For this review, take the finished solid that the model builds, in its own axes (mm). Face numbers are marked on the shaded views. A direction names the side the tool comes from. Give positions to 0.01 mm unless a question says otherwise; leave off trailing zeros. Loops run counter-clockwise (first coordinate to the right, second up) from the corner with the lowest first, then second, coordinate; pieces in that order, holes last. Notation, with made-up numbers: (66, 54.5) -> (113, 54.5) arc R12 cw to (113, 63.5) -> close; hole circle Ø2 at (66, -39). An arc over 180 degrees is marked (long way). Answer as CSV lines item,"result". Start each with the question number.
Item 1: Clearance check with a flat-ended pin moving along its axis: P1, Ø2, axis at x = -8, z = -39, coming from the -Y side. State where the tip first meets the part, or that it passes through.
Item 2: Machinability: for the marked faces 1 and 2, which of the approach directions +Z, -Z, +X, -X, +Y, -Y give a long, thin tool a straight path to every point of the face, cutting with its end or side? Answer none if there is none.
Item 3: Add section C-C on y = -5.5. State the section outline as (x, z) points.
Item 4: For L1, parallel to X at y = -2.25, z = 0; L2, parallel to Z at x = 0, y = -8.6, list the stretches that pass through material, from the lowest coordinate up. Write a range as from..to.
Item 5: Add section D-D on z = -42.5. State the section outline as (x, y) points, plus the area to 3 significant figures.
Item 6: Add section A-A on x = 0. State the section outline as (y, z) points, plus the area to 3 significant figures.
Item 7: Add section B-B on z = 0. State the section outline as (x, y) points, plus the area to 3 significant figures.
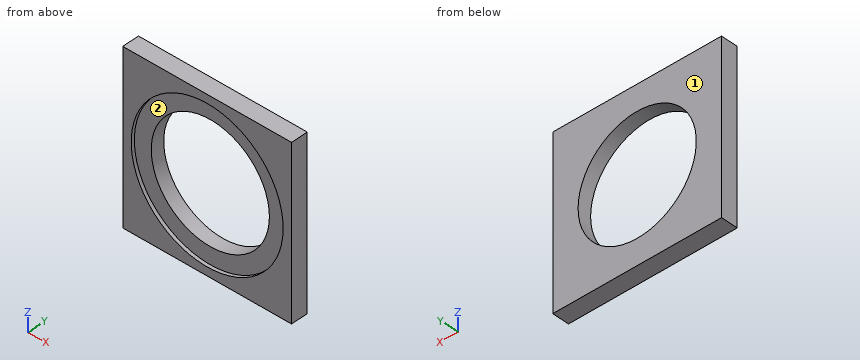
```python
from build123d import *

# Parameters (mm, degrees)
F0_W     = 100
F0_H     = 100
F0_R     = 35
F1_DEPTH = 10
F2_R     = 45
F3_DEPTH = 2


with BuildPart() as f1:
    # F0 (on Front) → F1 (new body)
    with BuildSketch(Plane.XZ):
        Rectangle(F0_W, F0_H)
        Circle(F0_R, mode=Mode.SUBTRACT)
    extrude(amount=F1_DEPTH)

    # F2 (on face) → F3 (cut)
    with BuildSketch(Plane.XZ.offset(10)):
        Circle(F2_R)
    extrude(amount=-F3_DEPTH, mode=Mode.SUBTRACT)


solid = f1.part
```
Computed values:
1,P1,"y = -8"
2,face 1,"+Z, -Z, +X, -X, +Y"
2,face 2,"-Y"
3,outline,"(-50, -50) -> (50, -50) -> (50, 50) -> (-50, 50) -> close; hole circle Ø70 at (0, 0)"
4,L1,"-50..-35, 35..50"
4,L2,"-50..-45, 45..50"
5,outline,"(-50, -10) -> (-14.79, -10) -> (-14.79, -8) -> (14.79, -8) -> (14.79, -10) -> (50, -10) -> (50, 0) -> (-50, 0) -> close"
5,area,"941 mm²"
6,outline,"(-10, -50) -> (0, -50) -> (0, -35) -> (-8, -35) -> (-8, -45) -> (-10, -45) -> close; (-10, 45) -> (-8, 45) -> (-8, 35) -> (0, 35) -> (0, 50) -> (-10, 50) -> close"
6,area,"260 mm²"
7,outline,"(-50, -10) -> (-45, -10) -> (-45, -8) -> (-35, -8) -> (-35, 0) -> (-50, 0) -> close; (35, -8) -> (45, -8) -> (45, -10) -> (50, -10) -> (50, 0) -> (35, 0) -> close"
7,area,"260 mm²"
